Input: part model. Units: mm. Frame: model coordinates. Face numbers are marked on the shaded views. A direction names the side the tool comes from. Round coordinates to 2 decimals unless told otherwise and drop trailing zeros. Write each loop counter-clockwise with the first axis right and the second up, starting at its lowest first coordinate (ties: lowest second). Pieces come first, ordered by that corner, then holes. Notation, with made-up numbers: (72.5, 27.25) - (129.5, 27.25) arc R32 ccw to (129.5, 61.25) - close; hole circle Ø11 at (4.5, -8.5). An arc over 180 degrees is marked (long way). One line per item, written item: value. Start each with the question number.
```python
from build123d import *

# Parameters (mm, degrees)
F2_R     = 2.5
F3_DEPTH = 5.001
F4_SIZE  = 1
F5_SIZE  = 0.5


with BuildPart() as f1:
    # F0 (on Front) → F1 (revolve)
    with BuildSketch(Plane.XZ):
        Polygon((-5, 24), (-5, 5), (0, 5), (20, 5), (20, 10), (0, 10), (0, 37), (-4, 37), (-4, 24), align=None)
    revolve(axis=Axis((1.734695, 0, 0), (1, 0, 0)))

    # F2 (on face) → F3 (cut, through all)
    with BuildSketch(Plane.YZ):
        with Locations((0, 29.5)):
            Circle(F2_R)
        with Locations((-25.547749, 14.75)):
            Circle(F2_R)
        with Locations((-25.547749, -14.75)):
            Circle(F2_R)
        with Locations((0, -29.5)):
            Circle(F2_R)
        with Locations((25.547749, -14.75)):
            Circle(F2_R)
        with Locations((25.547749, 14.75)):
            Circle(F2_R)
    extrude(amount=-F3_DEPTH, mode=Mode.SUBTRACT)

    # F4
    f4_edges = [f1.edges().sort_by_distance(p)[0] for p in [
        (20, 0, -10),
        (-4, 0, -37),
    ]]
    chamfer(f4_edges, length=F4_SIZE)

    # F5
    f5_edges = [f1.edges().sort_by_distance(p)[0] for p in [
        (-5, 0, -5),
        (20, 0, -5),
    ]]
    chamfer(f5_edges, length=F5_SIZE)


solid = f1.part
```
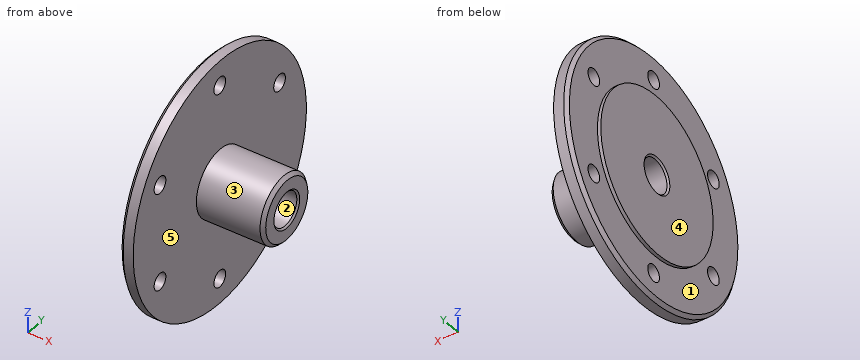
Q1. Pull-direction query (Z, two-part tool) for the marked faces 1, 2 and 3; classes: pulls with the +Z half, pulls with the -Z half, needs draft (parallel to the pull), parting line crosses it, or undercut.
Q2. Cut plane A-A, the plane y = 0. Count the separate pieces of the cut face and the enclosed holes in it, and give its area (4 significant figures).
Q3. Material intervals for probe 1 along Z at (x, y) = (-2.35, 0); probe 2 along Y at (x, z) = (-1.5, -12.5); probe 3 along Z at (x, y) = (1.5, 0), sorted ascending. Write a range as from..to.
Q4. Cut plane C-C, the plane x = -1.75. Output: boundary loops of the cut face in (y, z).
Q5. Access query for the marked faces 4 and 5. Directions: +Z, -Z, +X, -X, +Y, -Y. A direction counts if a zero-diameter tool reaches every point of the face in a straight line with its end or side. Return the directions, or none.
Q6. Contact query for flat-ended pins moving along their axis: pin 1 Ø8 at (y, z) = (0, 29.5) entering from -X; pin 2 Ø6 at (x, z) = (6, -14) entering from +Y; pin 3 Ø6.5 at (y, z) = (25.55, 14.75) entering from +X; pin 4 Ø8 at (x, z) = (9.5, 8) entering from +Y. Output: stop coordinate, or through.
Q7. Cut plane B-B, the plane z = 0. Output: boundary loops of the cut face in (x, y).
Q8. Cut plane D-D, the plane x = 11. Output: boundary loops of the cut face in (y, z), and give its area (3 significant figures).
A:
1. face 1: needs draft
1. face 2: undercut
1. face 3: parting line crosses it
2. separate pieces: 4
2. enclosed holes: 0
2. area: 451.5 mm²
3. probe 1: z = -37..-32, -27..-5, 5..27, 32..37
3. probe 2: y = -34.82..-26.64, -24.46..24.46, 26.64..34.82
3. probe 3: z = -10..-5, 5..10
4. outline: circle Ø74 at (0, 0); hole circle Ø5 at (-25.55, -14.75); hole circle Ø5 at (-25.55, 14.75); hole circle Ø10 at (0, 0); hole circle Ø5 at (0, -29.5); hole circle Ø5 at (0, 29.5); hole circle Ø5 at (25.55, -14.75); hole circle Ø5 at (25.55, 14.75)
5. face 4: +Z, -Z, -X, +Y, -Y
5. face 5: +X
6. pin 1: stops at x = -4
6. pin 2: passes through
6. pin 3: stops at x = 0
6. pin 4: stops at y = 9.17
7. outline: (-5, -24) - (-4, -24) - (-4, -36) - (-3, -37) - (0, -37) - (0, -10) - (19, -10) - (20, -9) - (20, -5.5) - (19.5, -5) - (-4.5, -5) - (-5, -5.5) - close; (-5, 5.5) - (-4.5, 5) - (19.5, 5) - (20, 5.5) - (20, 9) - (19, 10) - (0, 10) - (0, 37) - (-3, 37) - (-4, 36) - (-4, 24) - (-5, 24) - close
8. outline: circle Ø20 at (0, 0); hole circle Ø10 at (0, 0)
8. area: 236 mm²
